Check sheet for the modelled part. Datum: model origin and axes. Units: mm. Face numbers are marked on the shaded views. A direction names the side the tool comes from. Give positions to 0.01 mm unless a question says otherwise; leave off trailing zeros. Order: outer loops, then holes, each group sorted by start corner. A loop starts at its lowest first (then second) coordinate and runs counter-clockwise, first axis right, second up. Notation, with made-up numbers: M 28.5,48 L 59.5,48 A15 ccw 59.5,69 Z; hole C 57.25,41.5 d1. An arc over 180 degrees is marked long. One line per question, with ' | ' between items. Start each with the question number.
```python
from build123d import *

# Parameters (mm, degrees)
F0_W     = 450.85
F0_H     = 533.4
F1_DEPTH = 793.75
F2_W     = 406.4
F2_H     = 101.6
F2_H_2   = 177.8
F2_H_3   = 279.4
F3_DEPTH = 406.4


# Not quite as in the source:
# - a feature names something its author has since deleted; it is built from what else it names


with BuildPart() as f1:
    # F0 (on Top) → F1 (new body)
    with BuildSketch(Plane.XY):
        Rectangle(F0_W, F0_H)
    extrude(amount=-F1_DEPTH)

    # F2 (on face) → F3 (cut)
    with BuildSketch(Plane.XZ.offset(266.7)):
        with Locations((0, -95.25)):
            Rectangle(F2_W, F2_H)
        with Locations((0, -336.55)):
            Rectangle(F2_W, F2_H_2)
        with Locations((0, -628.65)):
            Rectangle(F2_W, F2_H_3)
    extrude(amount=-F3_DEPTH, mode=Mode.SUBTRACT)


solid = f1.part
```
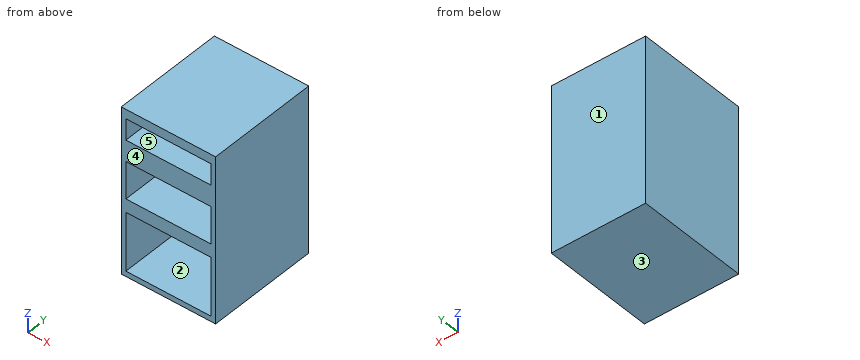
Item 1: Draft check along Z on the marked faces 3, 4 and 5. Enter one of: released by +Z, released by -Z, zero draft, split by the parting line, or undercut.
Item 2: Section check B-B, the plane x = 149. Record the cut outline in (y, z), then the cut area to 3 significant figures.
Item 3: Go/stop test with a flat-tipped pin: P1, Ø2, axis at x = 108, z = -125.5, coming from the -Y side. Record where the tip stops, or that it passes through.
Item 4: Section check A-A, the plane y = 33.5. Record the cut outline in (x, z) (3 decimals), then the cut area to 3 significant figures.
Item 5: Set-up check for the marked faces 1 and 2: record each of +Z, -Z, +X, -X, +Y, -Y from which the full face is reachable in a straight line by a thin tool's end or side.
Item 6: Scan lines: probe 1 along Z at (x, y) = (-25, 58); probe 2 along X at (y, z) = (-77.5, -390) (3 decimals); probe 3 along Y at (x, z) = (139, -528). Record each from-to range of solid material in increasing order. Write a range as [from, to].
Item 7: Section check C-C, the plane z = -272. Record the cut outline in (x, y) (3 decimals).
Reported:
1) face 3: released by -Z | face 4: zero draft | face 5: undercut
2) outline: M -266.7,-793.75 L 266.7,-793.75 L 266.7,0 L -266.7,0 L -266.7,-44.45 L 139.7,-44.45 L 139.7,-146.05 L -266.7,-146.05 L -266.7,-247.65 L 139.7,-247.65 L 139.7,-425.45 L -266.7,-425.45 L -266.7,-488.95 L 139.7,-488.95 L 139.7,-768.35 L -266.7,-768.35 Z | area: 196,000 mm^2
3) P1: stops at y = 139.7
4) outline: M -225.425,-793.75 L 225.425,-793.75 L 225.425,0 L -225.425,0 Z; hole M -203.2,-768.35 L 203.2,-768.35 L 203.2,-488.95 L -203.2,-488.95 Z; hole M -203.2,-425.45 L 203.2,-425.45 L 203.2,-247.65 L -203.2,-247.65 Z; hole M -203.2,-146.05 L 203.2,-146.05 L 203.2,-44.45 L -203.2,-44.45 Z | area: 131,000 mm^2
5) face 1: +Z, -Z, +X, -X, +Y | face 2: -Y
6) probe 1: z = [-793.75, -768.35], [-488.95, -425.45], [-247.65, -146.05], [-44.45, 0] | probe 2: x = [-225.425, -203.2], [203.2, 225.425] | probe 3: y = [139.7, 266.7]
7) outline: M -225.425,-266.7 L -203.2,-266.7 L -203.2,139.7 L 203.2,139.7 L 203.2,-266.7 L 225.425,-266.7 L 225.425,266.7 L -225.425,266.7 Z
